Drawing for the job (mm, zero at the part's lowest x, y, z). A direction names the side the tool comes from. Coordinates: 2 decimals unless noted, no trailing zeros. Write each loop counter-clockwise with the first axis right and the second up, starting at its lowest first coordinate (ties: lowest second). Pieces come first, ordered by that corner, then holes. Notation, with made-up numbers: M -32,29 L 1,29 A19 cw 1,40 Z; hole C 21,16 d3. An arc over 180 degrees is marked long. Use a Markdown table: item, result. Add a question column.
Q1. Pin check, flat tips, straight feed: pin 1 Ø22 at (x, y) = (41.5, 8.5) entering from -Z; pin 2 Ø2 at (x, z) = (41.5, 37) entering from +Y; pin 3 Ø23 at (x, y) = (50, 40) entering from -Z. Stop position of each tip, or through.
Q2. Slice it at D-D on x = 70.5. Write the cut outline in (y, z), then the cut area to 3 significant figures.
Q3. Mould opens along X. For the marked faces 1, 2, 3 and 4 say: released by +X, released by -X, zero draft, split by the parting line, or undercut.
Q4. Slice it at B-B on x = 50. Write the cut outline in (y, z).
Q5. Slice it at C-C on z = 56.5. Write the cut outline in (x, y), then the cut area to 3 significant figures.
Q6. Wall check: L1, parallel to X at y = 6, z = 13.5; L2, parallel to Y at x = 50, z = 54; L3, parallel to Z at x = 69.5, y = 38. Give the ranges that are in metal, low to high. Write a range as from..to.
Q7. Slice it at A-A on y = 40. Write the cut outline in (x, z).
Q8. Tool access for the marked faces 5, 6 and 7: list every direction of +Z, -Z, +X, -X, +Y, -Y with a clear straight run to the whole face (end or side of a thin tool).
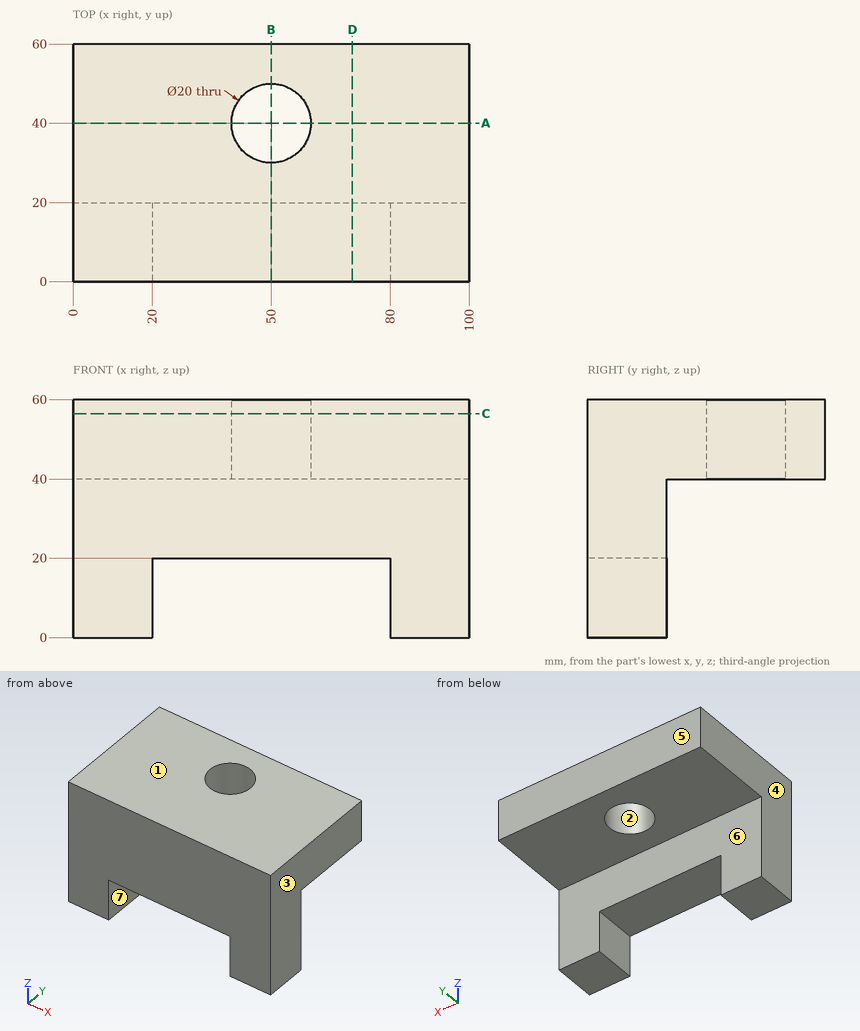
Recorded:
| question | item | result |
|---|---|---|
| 1 | pin 1 | z = 20 |
| 1 | pin 2 | y = 20 |
| 1 | pin 3 | z = 40 |
| 2 | outline | M 0,20 L 20,20 L 20,40 L 60,40 L 60,60 L 0,60 Z |
| 2 | area | 1,600 mm² |
| 3 | face 1 | zero draft |
| 3 | face 2 | undercut |
| 3 | face 3 | released by +X |
| 3 | face 4 | released by -X |
| 4 | outline | M 0,20 L 20,20 L 20,40 L 30,40 L 30,60 L 0,60 Z; M 50,40 L 60,40 L 60,60 L 50,60 Z |
| 5 | outline | M 0,0 L 100,0 L 100,60 L 0,60 Z; hole C 50,40 d20 |
| 5 | area | 5,690 mm² |
| 6 | L1 | 0..20, 80..100 |
| 6 | L2 | 0..30, 50..60 |
| 6 | L3 | 40..60 |
| 7 | outline | M 0,40 L 40,40 L 40,60 L 0,60 Z; M 60,40 L 100,40 L 100,60 L 60,60 Z |
| 8 | face 5 | +Z, -Z, +X, -X, +Y |
| 8 | face 6 | -Z, +X, -X, +Y |
| 8 | face 7 | -Z, +Y, -Y |
